Can you work these out from the model? Positions are in its coordinate system, mm. A direction names the side the tool comes from. Coordinates: 2 decimals unless noted, no trailing zeros. Write each loop counter-clockwise with the first axis right and the second up, starting at its lowest first coordinate (ties: lowest second). Pieces come first, ordered by that corner, then holes. Notation, with made-up numbers: M 40.25,-12 L 86.25,-12 A11 ccw 86.25,2 Z; hole C -6.5,-18.75 d5. An arc over 180 degrees is marked long. Answer as a JSON object with one key per item and string values. Group by question number.
from build123d import *

# Parameters (mm, degrees)
SKETCH1_W           = 12.3
SKETCH1_H           = 6
BOSS_EXTRUDE1_DEPTH = 7.7
SKETCH2_W           = 8.7
SKETCH2_H           = 4.6
CUT_EXTRUDE1_DEPTH  = 5
SKETCH3_W           = 1.1
SKETCH3_H           = 6
CUT_EXTRUDE2_DEPTH  = 4.4
SKETCH4_W           = 1.8
SKETCH4_H           = 0.7
CUT_EXTRUDE3_DEPTH  = 5
SKETCH5_W           = 10.1
SKETCH5_H           = 0.9
CUT_EXTRUDE4_DEPTH  = 4.4
SKETCH6_W           = 0.5
SKETCH6_H           = 0.5
BOSS_EXTRUDE2_DEPTH = 3.7


with BuildPart() as part:
    # Sketch1 → Boss-Extrude1 (new body)
    with BuildSketch(Plane(origin=(0, 0, 0), x_dir=(1, 0, 0), z_dir=(0, 1, 0))):
        Rectangle(SKETCH1_W, SKETCH1_H)
    extrude(amount=BOSS_EXTRUDE1_DEPTH)

    # Sketch2 → Cut-Extrude1 (cut)
    with BuildSketch(Plane(origin=(0, 7.7, 0), x_dir=(1, 0, 0), z_dir=(0, 1, 0))):
        Rectangle(SKETCH2_W, SKETCH2_H)
    extrude(amount=-CUT_EXTRUDE1_DEPTH, mode=Mode.SUBTRACT)

    # Sketch3 → Cut-Extrude2 (cut)
    with BuildSketch(Plane(origin=(0, 7.7, 0), x_dir=(1, 0, 0), z_dir=(0, 1, 0))):
        with Locations((-5.6, 0)):
            Rectangle(SKETCH3_W, SKETCH3_H)
        with Locations((5.6, 0)):
            Rectangle(SKETCH3_W, SKETCH3_H)
    extrude(amount=-CUT_EXTRUDE2_DEPTH, mode=Mode.SUBTRACT)

    # Sketch4 → Cut-Extrude3 (cut)
    with BuildSketch(Plane(origin=(0, 7.7, 0), x_dir=(1, 0, 0), z_dir=(0, 1, 0))):
        with Locations((-2.2, -2.65)):
            Rectangle(SKETCH4_W, SKETCH4_H)
        with Locations((2.2, -2.65)):
            Rectangle(SKETCH4_W, SKETCH4_H)
    extrude(amount=-CUT_EXTRUDE3_DEPTH, mode=Mode.SUBTRACT)

    # Sketch5 → Cut-Extrude4 (cut)
    with BuildSketch(Plane(origin=(0, 7.7, 0), x_dir=(1, 0, 0), z_dir=(0, 1, 0))):
        with Locations((0, -1.85)):
            Rectangle(SKETCH5_W, SKETCH5_H)
    extrude(amount=-CUT_EXTRUDE4_DEPTH, mode=Mode.SUBTRACT)

    # Sketch6 → Boss-Extrude2 (add)
    with BuildSketch(Plane(origin=(0, 2.7, 0), x_dir=(1, 0, 0), z_dir=(0, 1, 0))):
        with Locations((0, -1.15)):
            Rectangle(SKETCH6_W, SKETCH6_H)
        with Locations((-2.35, -1.15)):
            Rectangle(SKETCH6_W, SKETCH6_H)
        with Locations((2.35, -1.15)):
            Rectangle(SKETCH6_W, SKETCH6_H)
    extrude(amount=BOSS_EXTRUDE2_DEPTH)


solid = part.part
Q1. If we section it at C-C on x = 1: List the corners of the cut face in (y, z) for me.
Q2. If we section it at A-A on y = 3: List the corners of the cut face in (x, z) for me.
Q3. We'd pull the mould along X, two halves only. Please class faces 4 (the flat face through (0, 2.7, 0)), 5 (the flat face through (0, 5, -2.3)), 6 (the flat face through (5.05, 6, -1)), 7 (the flat face through (0, 4, -3)): pulls with the +X half, pulls with the -X half, needs draft (parallel to the pull), parting line crosses it, or undercut.
Q4. Will these pins go through, and if not, where does the flat tip stop? pin 1 (0.6 mm diameter, centred on y = 5, z = 2.5, fed in from -X); pin 2 (0.6 mm diameter, centred on x = 2.5, y = 3.5, fed in from +Z); pin 3 (0.6 mm diameter, centred on x = 2.5, z = 1, fed in from +Y).
Q5. On a 3-axis mill with a long thin cutter (end or side, diameter ignored), from which of +Z, -Z, +X, -X, +Y, -Y can I reach the whole of each face in a straight line? I mean faces 1 (the flat face through (-5.05, 6, -1)), 2 (the flat face through (0, 3, 3)), 3 (the flat face through (4.35, 5, 0)). Say none if no direction works.
Q6. Please list where these lines run through material, in increasing order: L1, parallel to Z at x = 2.5, y = 3.75; L2, parallel to Z at x = -1, y = 6; L3, parallel to Y at x = -3.5, z = 2.2.
Q7. If we section it at D-D on z = -1.8: List the corners of the cut face in (x, y) for me, and give its area (3 significant figures).
Q8. If we section it at B-B on y = 5.25: Give the number of separate pieces and of enclosed holes in the cut face, and give its area (4 significant figures).
Reply:
{
 "1": {"outline": "M 0,-3 L 7.7,-3 L 7.7,-2.3 L 2.7,-2.3 L 2.7,2.3 L 7.7,2.3 L 7.7,3 L 0,3 Z"},
 "2": {"outline": "M -6.15,-3 L 6.15,-3 L 6.15,3 L 3.1,3 L 3.1,2.3 L 4.35,2.3 L 4.35,-2.3 L -4.35,-2.3 L -4.35,2.3 L -3.1,2.3 L -3.1,3 L -6.15,3 Z; M -2.6,0.9 L -2.1,0.9 L -2.1,1.4 L -2.6,1.4 Z; M -1.3,2.3 L 1.3,2.3 L 1.3,3 L -1.3,3 Z; M -0.25,0.9 L 0.25,0.9 L 0.25,1.4 L -0.25,1.4 Z; M 2.1,0.9 L 2.6,0.9 L 2.6,1.4 L 2.1,1.4 Z"},
 "3": {"face 4": "undercut", "face 5": "undercut", "face 6": "pulls with the +X half", "face 7": "needs draft"},
 "4": {"pin 1": "x = -5.05", "pin 2": "z = 1.4", "pin 3": "y = 6.4"},
 "5": {"face 1": "+Z, -Z, -X, +Y", "face 2": "+Z, +X, -X, +Y, -Y", "face 3": "+Y"},
 "6": {"L1": "-3 to -2.3, 0.9 to 1.4", "L2": "-3 to -2.3, 2.3 to 3", "L3": "0 to 2.7"},
 "7": {"outline": "M -6.15,0 L 6.15,0 L 6.15,3.3 L 5.05,3.3 L 5.05,7.7 L 4.35,7.7 L 4.35,2.7 L -4.35,2.7 L -4.35,7.7 L -5.05,7.7 L -5.05,3.3 L -6.15,3.3 Z", "area": "41.5 mm^2"},
 "8": {"separate pieces": "7", "enclosed holes": "0", "area": "17.55 mm^2"}
}
